Could you check a few things on this model? Use its own coordinates, in mm. A direction names the side the tool comes from. Coordinates: 2 decimals unless noted, no trailing zeros. Loops run counter-clockwise (first coordinate to the right, second up) from the corner with the lowest first, then second, coordinate; pieces in that order, holes last.
from build123d import *

# Parameters (mm, degrees)
F0_R     = 7
F0_R_2   = 4.8
F1_DEPTH = 13
F2_W     = 6.828025
F2_H     = 5.5
F3_DEPTH = 8
F5_DEPTH = 12.5


with BuildPart() as f1:
    # F0 (on Top) → F1 (new body)
    with BuildSketch(Plane.XY):
        Circle(F0_R)
        Circle(F0_R_2, mode=Mode.SUBTRACT)
    extrude(amount=F1_DEPTH)

    # F2 (on Top) → F3 (cut)
    with BuildSketch(Plane.XY):
        with Locations((6.614012, 0)):
            Rectangle(F2_W, F2_H)
    extrude(amount=F3_DEPTH, mode=Mode.SUBTRACT)

    # F4 (on Front) → F5 (cut, symmetric)
    with BuildSketch(Plane.XZ):
        Polygon((3, 0), (6.5, 0), (6.5, 3.5), align=None)
    extrude(amount=F5_DEPTH, both=True, mode=Mode.SUBTRACT)


solid = f1.part
1) Imagine slicing it at D-D on y = 5. List the corners of the cut face in (x, z) for me.
2) For faces 4 (the flat face through (-2, -5, 13)), 5 (the flat face through (5, 2.75, 5)), which set-ups out of +Z, -Z, +X, -X, +Y, -Y let a thin tool reach every point of the face, with its end or its side?
3) We'd pull the mould along Y, two halves only. Please class faces 1 (the flat face through (4, -4, 1)), 2 (the cylindrical face through (-7, 0, 6)), 3 (the flat face through (5, -2.75, 5)): released by +Y, released by -Y, zero draft, split by the parting line, or undercut.
4) Imagine slicing it at C-C on z = 8.5. List the corners of the cut face in (x, y) for me, plus the area to 3 significant figures.
5) If I drill on L1, parallel to X at y = 0, z = 9.75; L2, parallel to Y at x = -3.25, z = 1.5, over which ranges is the centre line in solid material (lowest first)?
6) Will these pins go through, and if not, where does the flat tip stop? pin 1 (1.3 mm diameter, centred on x = 5.5, z = 5, fed in from -Y); pin 2 (4 mm diameter, centred on x = 4, z = 10.5, fed in from -Y); pin 3 (2 mm diameter, centred on x = 5, z = 5, fed in from +Y).
7) Imagine slicing it at A-A on x = 0. List the corners of the cut face in (y, z) for me.
8) Imagine slicing it at B-B on y = 0. List the corners of the cut face in (x, z) for me.
Solved:
1. outline: (-4.9, 0) - (3, 0) - (4.9, 1.9) - (4.9, 13) - (-4.9, 13) - close
2. face 4: +Z, +X, -X, +Y, -Y
2. face 5: -Z, +X
3. face 1: zero draft
3. face 2: split by the parting line
3. face 3: undercut
4. outline: circle Ø14 at (0, 0); hole circle Ø9.6 at (0, 0)
4. area: 81.6 mm2
5. L1: x = -7 to -4.8, 4.8 to 7
5. L2: y = -6.2 to -3.53, 3.53 to 6.2
6. pin 1: stops at y = -5.05
6. pin 2: stops at y = -6.71
6. pin 3: stops at y = 5.74
7. outline: (-7, 0) - (-4.8, 0) - (-4.8, 13) - (-7, 13) - close; (4.8, 0) - (7, 0) - (7, 13) - (4.8, 13) - close
8. outline: (-7, 0) - (-4.8, 0) - (-4.8, 13) - (-7, 13) - close; (4.8, 8) - (7, 8) - (7, 13) - (4.8, 13) - close
